Check sheet for the modelled part. Datum: model origin and axes. Units: mm. Face numbers are marked on the shaded views. A direction names the side the tool comes from. Give positions to 0.01 mm unless a question says otherwise; leave off trailing zeros.
Item 1: Material ranges on line 1 along Y through (x, z) = (-22.5, -3.85) (3 decimals); line 2 along X through (y, z) = (-21, -89); line 3 along Y through (x, z) = (-1, -17), recorded low to high.
Item 2: Gauge pin test, flat ends, axial feed: P1, Ø3, axis at x = -23.5, y = 39.5, coming from the -Z side; P2, Ø6, axis at x = -13, y = 42, coming from the +Z side; P3, Ø3, axis at x = -23.5, z = -12, coming from the -Y side. Record the tip position at first contact, or that the pin passes through.
Item 3: Access from +Z, -Z, +X, -X, +Y, -Y to the whole of each face (thin tool, end or side, straight path). Record for the marked faces 1, 2 and 3.
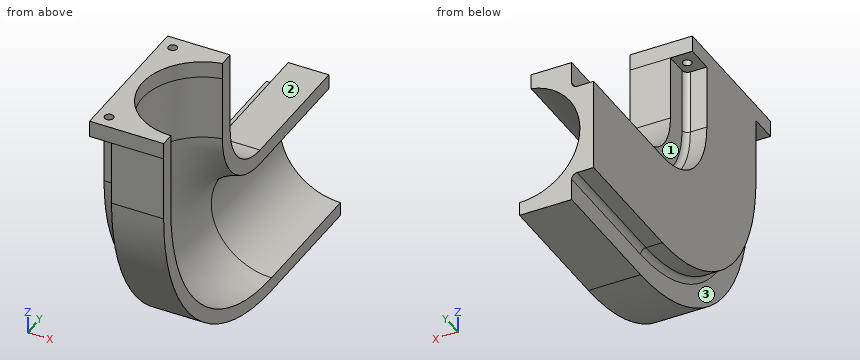
from build123d import *

# Parameters (mm, degrees)
EXTRUDE_1_DEPTH     = 6
SKETCH_4_R          = 1.605
CUT_EXTRUDE_1_DEPTH = 10
SWEEP_START         = -4.2
SWEEP_1_2_DEPTH     = 4.2


# Read off the part's stored shape, not the designer's step: 切除-扫描1
with BuildPart() as part:
    # 草图1 → 凸台-拉伸1 (new body)
    with BuildSketch(Plane.XY):
        with BuildLine():
            Line((0, 0), (-27, 0))
            Line((-27, 0), (-27, -54))
            Line((-27, -54), (0, -54))
            Line((0, -54), (0, -49))
            ThreePointArc((0, -49), (-22, -27), (0, -5))
            Line((0, -5), (0, 0))
        make_face()
    extrude(amount=-EXTRUDE_1_DEPTH)

    # Sweep 1: sweep along a path in 草图3
    with BuildLine(Plane(origin=(0, 0, 0), x_dir=(0, 0, -1), z_dir=(1, 0, 0))) as sweep_1_path:
        Line((6, -27), (29.659999985, -27.000851338))
        ThreePointArc((29.659999985, -27.000851338), (63.354746468, -13.045095672), (77.311714535, 20.649148631))
        Line((77.311714535, 20.649148631), (77.311714535, 68.299148631))
    # 草图2 → Sweep 1 (sweep)
    with BuildSketch(Plane(origin=(0, 0, -6), x_dir=(-1, 0, 0), z_dir=(0, 0, -1))):
        with BuildLine():
            Line((19, 0), (19, -8))
            ThreePointArc((19, -8), (19.585786438, -9.414213562), (21, -10))
            Line((21, -10), (27, -10))
            Line((27, -10), (27, -44))
            Line((27, -44), (21, -44))
            ThreePointArc((21, -44), (19.585786438, -44.585786438), (19, -46))
            Line((19, -46), (19, -54))
            Line((19, -54), (0, -54))
            Line((0, -54), (0, -49))
            ThreePointArc((0, -49), (22, -27), (0, -5))
            Line((0, -5), (0, 0))
            Line((0, 0), (19, 0))
        make_face()
    sweep(path=sweep_1_path.line)

    # 草图4 → 切除-拉伸1 (cut)
    with BuildSketch(Plane(origin=(0, 0, -6), x_dir=(-1, 0, 0), z_dir=(0, 0, -1))):
        with Locations((22.5, -5)):
            Circle(SKETCH_4_R)
    cut_extrude_1 = extrude(amount=-CUT_EXTRUDE_1_DEPTH, mode=Mode.SUBTRACT)

    # 镜向1: 切除-拉伸1 across plane
    add(cut_extrude_1.mirror(Plane.ZX.offset(-27)), mode=Mode.SUBTRACT)

    # Sweep 1 2 outline → Sweep 1 2 (cut)
    with BuildSketch(Plane.YZ.offset(SWEEP_START)):
        with BuildLine():
            Line((-0.000851338, -29.659999985), (0, -6))
            Line((0, -6), (0, 1))
            Line((0, 1), (-7, 1))
            Line((-7, 1), (-7, -57))
            Line((-7, -57), (68.298417771, -57))
            Line((68.298417771, -57), (68.298177112, -50.311714553))
            Line((68.298177112, -50.311714553), (20.648177112, -50.311714553))
            ThreePointArc((20.648177112, -50.311714553), (6.046443933, -44.262519896), (-0.000851338, -29.659999985))
        make_face()
    extrude(amount=SWEEP_1_2_DEPTH, mode=Mode.SUBTRACT)


solid = part.part
Report:
1. line 1: y = -54 to -50.605, -47.395 to -6.605, -3.395 to 0
1. line 2: x = -19 to 0
1. line 3: y = -54 to -48.98
2. P1: stops at z = -94.31
2. P2: stops at z = -50.31
2. P3: stops at y = -44
3. face 1: -X, +Y
3. face 2: +Z, +X, -X, +Y
3. face 3: -Z, -X, -Y
